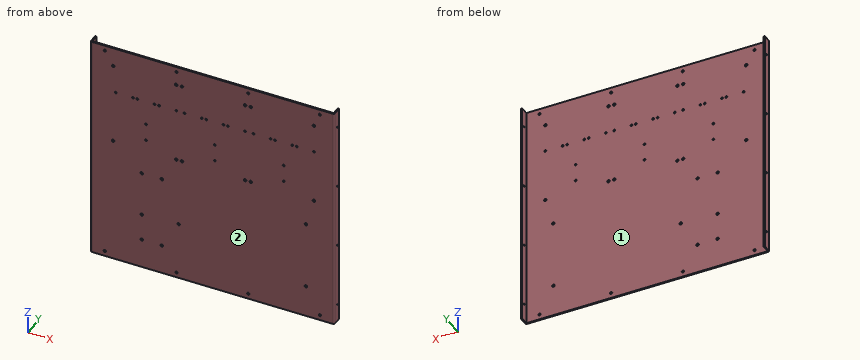
from build123d import *

# Parameters (mm, degrees)
BASE_FLANGE3_DEPTH  = 406.4
SKETCH10_R          = 1.4478
CUT_EXTRUDE3_DEPTH  = 594.198769469
SKETCH11_R          = 2.032
CUT_EXTRUDE4_DEPTH  = 594.139546967
CUT_EXTRUDE10_START = 2.286
SKETCH13_R          = 1.651
SKETCH13_R_2        = 2.286
CUT_EXTRUDE10_DEPTH = 2.286
SKETCH14_R          = 2.286
CUT_EXTRUDE11_DEPTH = 2.286


# Sheet-metal steps are written as plain solids
with BuildPart() as part:
    # Sketch1 → Base-Flange3 (new body)
    with BuildSketch(Plane.XY):
        with BuildLine():
            Line((431.8, 16.51), (431.8, 2.4384))
            ThreePointArc((431.8, 2.4384), (431.085809175, 0.714190825), (429.3616, 0))
            Line((429.3616, 0), (2.4384, 0))
            ThreePointArc((2.4384, 0), (0.714190825, 0.714190825), (0, 2.4384))
            Line((0, 2.4384), (0, 16.51))
            Line((0, 16.51), (2.286, 16.51))
            Line((2.286, 16.51), (2.286, 2.4384))
            ThreePointArc((2.286, 2.4384), (2.330636927, 2.330636927), (2.4384, 2.286))
            Line((2.4384, 2.286), (429.3616, 2.286))
            ThreePointArc((429.3616, 2.286), (429.469363073, 2.330636927), (429.514, 2.4384))
            Line((429.514, 2.4384), (429.514, 16.51))
            Line((429.514, 16.51), (431.8, 16.51))
        make_face()
    extrude(amount=BASE_FLANGE3_DEPTH)

    # Sketch10 → Cut-Extrude3 (cut, through all)
    with BuildSketch(Plane(origin=(431.8, 0, 0), x_dir=(0, 0, -1), z_dir=(1, 0, 0))):
        with Locations((-31.75, 10.16)):
            Circle(SKETCH10_R)
        with Locations((-146.05, 10.16)):
            Circle(SKETCH10_R)
        with Locations((-260.35, 10.16)):
            Circle(SKETCH10_R)
        with Locations((-374.65, 10.16)):
            Circle(SKETCH10_R)
    extrude(amount=-CUT_EXTRUDE3_DEPTH, mode=Mode.SUBTRACT)

    # Sketch11 → Cut-Extrude4 (cut, through all)
    with BuildSketch(Plane(origin=(0, 2.286, 0), x_dir=(-1, 0, 0), z_dir=(0, 1, 0))):
        with Locations(Location((-406.4, 397.002, 0), (0, 0, 90))):
            Circle(SKETCH11_R)
        with Locations(Location((-279.4, 397.002, 0), (0, 0, 90))):
            Circle(SKETCH11_R)
        with Locations(Location((-152.4, 397.002, 0), (0, 0, 90))):
            Circle(SKETCH11_R)
        with Locations(Location((-25.4, 397.002, 0), (0, 0, 90))):
            Circle(SKETCH11_R)
        with Locations(Location((-406.4, 9.398, 0), (0, 0, 90))):
            Circle(SKETCH11_R)
        with Locations(Location((-279.4, 9.398, 0), (0, 0, 90))):
            Circle(SKETCH11_R)
        with Locations(Location((-152.4, 9.398, 0), (0, 0, 90))):
            Circle(SKETCH11_R)
        with Locations(Location((-25.4, 9.398, 0), (0, 0, 90))):
            Circle(SKETCH11_R)
    extrude(amount=-CUT_EXTRUDE4_DEPTH, mode=Mode.SUBTRACT)

    # Sketch13 → Cut-Extrude10 (cut)
    with BuildSketch(Plane(origin=(13.91994535, 0, 411.979952645), x_dir=(0, 0, -1), z_dir=(0, 1, 0)).offset(CUT_EXTRUDE10_START)):
        with Locations(Location((89.98703359, -313.064950531, 0), (0, 0, 180))):
            Circle(SKETCH13_R)
        with Locations(Location((89.98703359, -343.544950531, 0), (0, 0, 180))):
            Circle(SKETCH13_R)
        with Locations(Location((89.98703359, -274.710950531, 0), (0, 0, 180))):
            Circle(SKETCH13_R)
        with Locations(Location((89.98703359, -305.190950531, 0), (0, 0, 180))):
            Circle(SKETCH13_R)
        with Locations(Location((89.98703359, -351.418950531, 0), (0, 0, 180))):
            Circle(SKETCH13_R)
        with Locations(Location((89.98703359, -381.898950531, 0), (0, 0, 180))):
            Circle(SKETCH13_R)
        with Locations(Location((133.92903359, -328.304950531, 0), (0, 0, 180))):
            Circle(SKETCH13_R)
        with Locations(Location((164.40903359, -328.304950531, 0), (0, 0, 180))):
            Circle(SKETCH13_R)
        with Locations(Location((39.94903359, -381.898950531, 0), (0, 0, 180))):
            Circle(SKETCH13_R_2)
        with Locations(Location((184.72903359, -381.898950531, 0), (0, 0, 180))):
            Circle(SKETCH13_R_2)
        with Locations(Location((39.94903359, -270.138950531, 0), (0, 0, 180))):
            Circle(SKETCH13_R_2)
        with Locations(Location((184.72903359, -270.138950531, 0), (0, 0, 180))):
            Circle(SKETCH13_R_2)
        with Locations(Location((89.98703359, -191.144950531, 0), (0, 0, 180))):
            Circle(SKETCH13_R)
        with Locations(Location((89.98703359, -221.624950531, 0), (0, 0, 180))):
            Circle(SKETCH13_R)
        with Locations(Location((89.98703359, -152.790950531, 0), (0, 0, 180))):
            Circle(SKETCH13_R)
        with Locations(Location((89.98703359, -183.270950531, 0), (0, 0, 180))):
            Circle(SKETCH13_R)
        with Locations(Location((89.98703359, -229.498950531, 0), (0, 0, 180))):
            Circle(SKETCH13_R)
        with Locations(Location((89.98703359, -259.978950531, 0), (0, 0, 180))):
            Circle(SKETCH13_R)
        with Locations(Location((133.92903359, -206.384950531, 0), (0, 0, 180))):
            Circle(SKETCH13_R)
        with Locations(Location((164.40903359, -206.384950531, 0), (0, 0, 180))):
            Circle(SKETCH13_R)
        with Locations(Location((39.94903359, -259.978950531, 0), (0, 0, 180))):
            Circle(SKETCH13_R_2)
        with Locations(Location((184.72903359, -259.978950531, 0), (0, 0, 180))):
            Circle(SKETCH13_R_2)
        with Locations(Location((39.94903359, -148.218950531, 0), (0, 0, 180))):
            Circle(SKETCH13_R_2)
        with Locations(Location((184.72903359, -148.218950531, 0), (0, 0, 180))):
            Circle(SKETCH13_R_2)
        with Locations(Location((89.98703359, -69.224950531, 0), (0, 0, 180))):
            Circle(SKETCH13_R)
        with Locations(Location((89.98703359, -99.704950531, 0), (0, 0, 180))):
            Circle(SKETCH13_R)
        with Locations(Location((89.98703359, -30.870950531, 0), (0, 0, 180))):
            Circle(SKETCH13_R)
        with Locations(Location((89.98703359, -61.350950531, 0), (0, 0, 180))):
            Circle(SKETCH13_R)
        with Locations(Location((89.98703359, -107.578950531, 0), (0, 0, 180))):
            Circle(SKETCH13_R)
        with Locations(Location((89.98703359, -138.058950531, 0), (0, 0, 180))):
            Circle(SKETCH13_R)
        with Locations(Location((133.92903359, -84.464950531, 0), (0, 0, 180))):
            Circle(SKETCH13_R)
        with Locations(Location((164.40903359, -84.464950531, 0), (0, 0, 180))):
            Circle(SKETCH13_R)
        with Locations(Location((39.94903359, -138.058950531, 0), (0, 0, 180))):
            Circle(SKETCH13_R_2)
        with Locations(Location((184.72903359, -138.058950531, 0), (0, 0, 180))):
            Circle(SKETCH13_R_2)
        with Locations(Location((39.94903359, -26.298950531, 0), (0, 0, 180))):
            Circle(SKETCH13_R_2)
        with Locations(Location((184.72903359, -26.298950531, 0), (0, 0, 180))):
            Circle(SKETCH13_R_2)
    extrude(amount=-CUT_EXTRUDE10_DEPTH, mode=Mode.SUBTRACT)

    # Sketch14 → Cut-Extrude11 (cut)
    with BuildSketch(Plane(origin=(0, 2.286, 0), x_dir=(1, 0, 0), z_dir=(0, 1, 0))):
        with Locations(Location((156.154345185, -103.963043442, 0), (0, 0, 270))):
            Circle(SKETCH14_R)
        with Locations(Location((381.687370192, -56.973043442, 0), (0, 0, 270))):
            Circle(SKETCH14_R)
        with Locations(Location((381.687370192, -177.369043442, 0), (0, 0, 270))):
            Circle(SKETCH14_R)
        with Locations(Location((126.436345185, -181.077443442, 0), (0, 0, 270))):
            Circle(SKETCH14_R)
        with Locations(Location((90.876345185, -181.077443442, 0), (0, 0, 270))):
            Circle(SKETCH14_R)
        with Locations(Location((90.876345185, -101.067443442, 0), (0, 0, 270))):
            Circle(SKETCH14_R)
        with Locations(Location((90.876345185, -52.807443442, 0), (0, 0, 270))):
            Circle(SKETCH14_R)
        with Locations(Location((126.436345185, -52.807443442, 0), (0, 0, 270))):
            Circle(SKETCH14_R)
    extrude(amount=-CUT_EXTRUDE11_DEPTH, mode=Mode.SUBTRACT)


solid = part.part
Input: part model. Units: mm. Frame: model coordinates. Face numbers are marked on the shaded views. A direction names the side the tool comes from. Coordinates: 2 decimals unless noted, no trailing zeros. Loops run counter-clockwise (first coordinate to the right, second up) from the corner with the lowest first, then second, coordinate; pieces in that order, holes last. Notation, with made-up numbers: (-29.5, 29) -> (4.5, 29) arc R24 ccw to (4.5, 39) -> close; hole circle Ø5 at (-10.75, -31.75). An arc over 180 degrees is marked (long way). Write item = value, one per line. Start each with the question number.
Item 1: Cut plane A-A, the plane y = 5.25. Return loops of the section in (x, z), plus the area to 3 significant figures.
Item 2: Reachability of the marked faces 1 and 2 from +Z, -Z, +X, -X, +Y, -Y: full face, straight path, thin tool, end or side. Return the list, or none.
Item 3: Cut plane C-C, the plane x = 137.5. Return loops of the section in (y, z), plus the area to 3 significant figures.
Item 4: Cut plane B-B, the plane z = 335. Return loops of the section in (x, y), plus the area to 3 significant figures.
Item 5: First-contact query: P1, Ø1.5, axis at y = 12.5, z = 300, coming from the -X side; P2, Ø4, axis at x = 319.11, z = 321.99, coming from the +Y side. Flat tips, straight axial feed; report the tip coordinate or a pass-through.
Item 6: Material intervals for line 1 (X direction, y = 14.25, z = 303); line 2 (Z direction, x = 279.4, y = 0.5); line 3 (Y direction, x = 324, z = 288), sorted ascending.
Ans:
q1.outline = (0, 0) -> (2.29, 0) -> (2.29, 406.4) -> (0, 406.4) -> close; (429.51, 0) -> (431.8, 0) -> (431.8, 406.4) -> (429.51, 406.4) -> close
q1.area = 1,860 mm²
q2.face_1 = +Z, -Z, +Y
q2.face_2 = +Z, -Z, +X, -X, -Y
q3.outline = (0, 0) -> (2.29, 0) -> (2.29, 406.4) -> (0, 406.4) -> close
q3.area = 929 mm²
q4.outline = (0, 2.44) arc R2.44 ccw to (2.44, 0) -> (429.36, 0) arc R2.44 ccw to (431.8, 2.44) -> (431.8, 16.51) -> (429.51, 16.51) -> (429.51, 2.44) arc R0.15 cw to (429.36, 2.29) -> (2.44, 2.29) arc R0.15 cw to (2.29, 2.44) -> (2.29, 16.51) -> (0, 16.51) -> close
q4.area = 1,050 mm²
q5.P1 = 0
q5.P2 = 2.29
q6.line_1 = 0 to 2.29, 429.51 to 431.8
q6.line_2 = 0 to 7.37, 11.43 to 394.97, 399.03 to 406.4
q6.line_3 = 0 to 2.29
